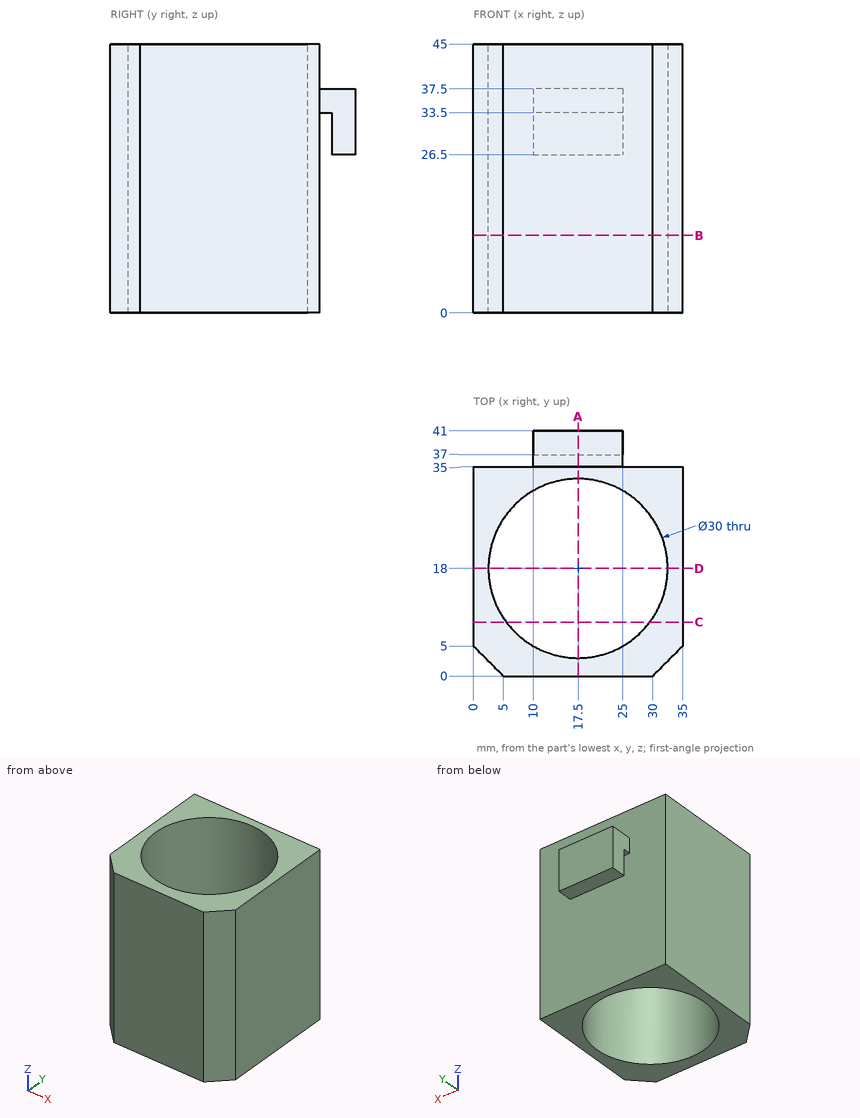
Part print with two shaded views. Sizes in mm from the minimum x, y, z corner. Round coordinates to 2 decimals unless told otherwise and drop trailing zeros. Order: outer loops, then holes, each group sorted by start corner. A loop starts at its lowest first (then second) coordinate and runs counter-clockwise, first axis right, second up. Notation, with made-up numbers: M -36,56 L -11,56 A22 cw -11,70 Z; hole C 52,27 d3. An arc over 180 degrees is marked long. Put each result on its own line as item: value. Start each with the question number.
1. Drop flat-ended pins along their axis: pin 1 (5 mm diameter, centred on y = 38, z = 31.5, fed in from +X); pin 2 (1 mm diameter, centred on x = 5, z = 5, fed in from +Y); pin 3 (0.6 mm diameter, centred on x = 15, y = 36, fed in from -Z). Give the stop position or say it passes through.
2. Drill centre lines: probe 1 along Y at (x, z) = (17, 33); probe 2 along Y at (x, z) = (17.5, 11.5); probe 3 along Y at (x, z) = (2, 15). Where is each one in solid material? Low to high. Write a range as [from, to].
3. Slice it at D-D on y = 18. List the corners of the cut face in (x, z), then the cut area to 3 significant figures.
4. Slice it at B-B on z = 13. List the corners of the cut face in (x, y), then the cut area to 3 significant figures.
5. Slice it at C-C on y = 9. List the corners of the cut face in (x, z), then the cut area to 3 significant figures.
6. Slice it at A-A on x = 17.5. List the corners of the cut face in (y, z), then the cut area to 3 significant figures.
Findings:
1. pin 1: x = 25
1. pin 2: y = 35
1. pin 3: z = 33.5
2. probe 1: [0, 3.01], [32.99, 35], [37, 41]
2. probe 2: [0, 3], [33, 35]
2. probe 3: [3, 35]
3. outline: M 0,0 L 2.5,0 L 2.5,45 L 0,45 Z; M 32.5,0 L 35,0 L 35,45 L 32.5,45 Z
3. area: 225 mm2
4. outline: M 0,5 L 5,0 L 30,0 L 35,5 L 35,35 L 0,35 Z; hole C 17.5,18 d30
4. area: 493 mm2
5. outline: M 0,0 L 5.5,0 L 5.5,45 L 0,45 Z; M 29.5,0 L 35,0 L 35,45 L 29.5,45 Z
5. area: 495 mm2
6. outline: M 0,0 L 3,0 L 3,45 L 0,45 Z; M 33,0 L 35,0 L 35,33.5 L 37,33.5 L 37,26.5 L 41,26.5 L 41,37.5 L 35,37.5 L 35,45 L 33,45 Z
6. area: 277 mm2
